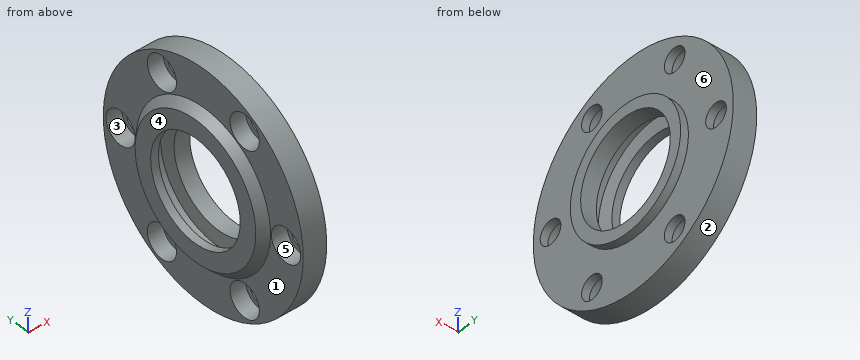
from build123d import *

# Parameters (mm, degrees)
SKETCH_1_W                = 6
SKETCH_1_H                = 29
SKETCH_2_R                = 19.5
EXTRUDE_1_DEPTH           = 2
EXTRUDE_1_TAPER           = 45
SKETCH_3_R                = 16
EXTRUDE_2_DEPTH           = 2
HOLE_WIZARD_1_D           = 6
HOLE_WIZARD_1_DEPTH       = 8
HOLE_WIZARD_1_CBORE_D     = 8.5
HOLE_WIZARD_1_CBORE_DEPTH = 4


with BuildPart() as part:
    # Эскиз1 → Повернуть1 (revolve)
    with BuildSketch(Plane.XY, mode=Mode.PRIVATE) as revolve_1_sk:
        with Locations((5, 14.5)):
            Rectangle(SKETCH_1_W, SKETCH_1_H)
    revolve(revolve_1_sk.sketch.rotate(Axis((2, 0, 0), (1, 0, 0)), 270), axis=Axis((2, 0, 0), (1, 0, 0)))

    # Эскиз2 → Бобышка-Вытянуть1 (add)
    with BuildSketch(Plane.ZY.offset(-2)):
        Circle(SKETCH_2_R)
    extrude(amount=EXTRUDE_1_DEPTH, taper=EXTRUDE_1_TAPER)

    # Эскиз3 → Бобышка-Вытянуть2 (add)
    with BuildSketch(Plane(origin=(8, 0, 0), x_dir=(0, 0, -1), z_dir=(1, 0, 0))):
        Circle(SKETCH_3_R)
    extrude(amount=EXTRUDE_2_DEPTH)

    # Эскиз4 → Вырез-Повернуть1 (revolve, cut)
    with BuildSketch(Plane(origin=(0, 0, 0), x_dir=(-1, 0, 0), z_dir=(0, 0, -1)), mode=Mode.PRIVATE) as cut_revolve_1_sk:
        Polygon((-10, 13), (-10, 0), (0, 0), (0, 13), (-2, 13), (-2.5, 16.373590872), (-5.5, 16.373590872), (-6, 13), align=None)
    revolve(cut_revolve_1_sk.sketch.rotate(Axis((10, 0, 0), (-1, 0, 0)), 270), axis=Axis((10, 0, 0), (-1, 0, 0)), mode=Mode.SUBTRACT)

    # Отверстие1
    with Locations(Plane.ZY.offset(-2)):
        with Locations((20.784609691, -12), (0, -24), (-20.784609691, -12), (-20.784609691, 12), (0, 24), (20.784609691, 12)):
            CounterBoreHole(HOLE_WIZARD_1_D / 2, HOLE_WIZARD_1_CBORE_D / 2, HOLE_WIZARD_1_CBORE_DEPTH, depth=HOLE_WIZARD_1_DEPTH)


solid = part.part
Build history of the part. All positions in model axes, mm. Face numbers are marked on the shaded views. A direction names the side the tool comes from. Give positions to 0.01 mm unless a question says otherwise; leave off trailing zeros. Order: outer loops, then holes, each group sorted by start corner. A loop starts at its lowest first (then second) coordinate and runs counter-clockwise, first axis right, second up. Notation, with made-up numbers: M 43,53.25 L 93,53.25 A10 cw 93,57.25 Z; hole C 70,49.25 d5. An arc over 180 degrees is marked long. Put each result on its own line as item: value.
Item 1: Two-plate mould, pull along Z, no slides. Class the marked faces 1, 2 and 3: +Z half, -Z half, draft (parallel to the pull), parting line (faces both ways), or undercut.
From the geometry:
face 1: draft
face 2: parting line
face 3: undercut
Item 2: Slice it at B-B, the plane x = 9. Write the cut outline in (y, z), plus the area to 3 significant figures.
From the geometry:
outline: C 0,0 d32; hole C 0,0 d26
area: 273 mm2
Item 3: Flat gauge pins, fed straight in: pin 1 Ø13.5 at (y, z) = (-12, -20.78) entering from +X; pin 2 Ø5 at (x, z) = (1, -2.5) entering from -Y; pin 3 Ø7 at (y, z) = (-24, 0) entering from -X. Where does each tip first touch, or does it go through?
From the geometry:
pin 1: stops at x = 8
pin 2: stops at y = -29
pin 3: stops at x = 6
Item 4: 3-axis set-ups, long thin cutter, end or side, ignore diameter. For the marked faces 4, 5 and 6: which of +Z, -Z, +X, -X, +Y, -Y reach the whole face in a straight line?
From the geometry:
face 4: +Z, -Z, -X, +Y, -Y
face 5: -X
face 6: +X
Item 5: Slice it at C-C, the plane y = -14. Give the number of separate pieces and of enclosed holes in the cut face, plus the area to 3 significant figures.
From the geometry:
separate pieces: 3
enclosed holes: 1
area: 247 mm2
Item 6: Slice it at A-A, the plane y = 22. Write the cut outline in (x, z), plus the area to 3 significant figures.
From the geometry:
outline: M 2,-18.89 L 8,-18.89 L 8,-2.24 L 6,-2.24 L 6,-3.75 L 2,-3.75 Z; M 2,3.75 L 6,3.75 L 6,2.24 L 8,2.24 L 8,18.89 L 2,18.89 Z
area: 188 mm2
Item 7: Probe line 1 (Y direction, x = 3.55, z = 0); line 2 (Y direction, x = 4.5, z = -21.5); line 3 (X direction, y = 12.5, z = 12). List the from-to ranges inside material, lowest first. Write a range as [from, to].
From the geometry:
line 1: y = [-29, -28.25], [-19.75, -16.37], [16.37, 19.75], [28.25, 29]
line 2: y = [-19.46, -16.19], [-7.81, 7.81], [16.19, 19.46]
line 3: x = [0, 8]
